Verification items for the finished model (mm, model axes). Face numbers are marked on the shaded views. A direction names the side the tool comes from. Give positions to 0.01 mm unless a question says otherwise; leave off trailing zeros. Write each loop counter-clockwise with the first axis right and the second up, starting at its lowest first coordinate (ties: lowest second). Pieces come first, ordered by that corner, then holes. Notation, with made-up numbers: (79.25, 80.25) -> (117.25, 80.25) arc R14 ccw to (117.25, 104.25) -> close; hole circle Ø10 at (-29.5, 52). An arc over 180 degrees is marked (long way). Answer as CSV lines item,"result". Start each with the question number.
1) Sectioned sample at A-A on y = 0. Give the number of separate pieces and of enclosed holes in the cut face, and give its area (3 significant figures).
2) Gauge pin test, flat ends, axial feed: pin 1 Ø3 at (x, z) = (-98, 45.5) entering from +Y; pin 2 Ø2.5 at (y, z) = (-0.5, 28) entering from +X; pin 3 Ø1.5 at (y, z) = (-4.5, 22.5) entering from +X; pin 4 Ø18.5 at (x, z) = (-110, 33) entering from -Y. Record the tip position at first contact, or that the pin passes through.
3) Sectioned sample at B-B on x = 0. Record the cut outline in (y, z).
4) Mould release check, pull along Z, two halves, no side actions. Record for the marked faces 1 and 2: released by +Z, released by -Z, zero draft, split by the parting line, or undercut.
5) Sectioned sample at D-D on z = 58. Record the cut outline in (x, y), and give its area (3 significant figures).
6) Material ranges on L1, parallel to X at y = 2, z = 34.5; L2, parallel to X at y = -1.5, z = 34.5; L3, parallel to Z at x = -29.5, y = -1.25, recorded low to high.
7) Tool access check on the marked faces 3, 4, 5 and 6. Record the directions out of +Z, -Z, +X, -X, +Y, -Y that give a thin tool (end or side, any length) a straight path to the whole face; none if there is none.
```python
from build123d import *

# Parameters (mm, degrees)
SKETCH1_R           = 6.35
SKETCH1_R_2         = 3.175
BOSS_EXTRUDE1_DEPTH = 62.992
SKETCH3_R           = 3.175
SKETCH6_W           = 22.86
SKETCH6_H           = 1.5875
BOSS_EXTRUDE3_DEPTH = 29.21
SKETCH7_R           = 4.7625
CUT_EXTRUDE1_DEPTH  = 29.21
SKETCH9_R           = 6.35
SKETCH9_R_2         = 3.175
BOSS_EXTRUDE5_DEPTH = 6.35
SKETCH10_R          = 6.35
SKETCH10_R_2        = 5.55625
CUT_EXTRUDE6_DEPTH  = 12.7
SKETCH12_R          = 6.35
SKETCH12_R_2        = 5.55625
CUT_EXTRUDE7_DEPTH  = 12.7
SKETCH13_R          = 5.55625
SKETCH13_R_2        = 3.175
CUT_EXTRUDE8_DEPTH  = 6.35
SKETCH14_R          = 5.55625
SKETCH14_R_2        = 3.175
CUT_EXTRUDE9_DEPTH  = 6.35
SKETCH16_R          = 3.96875
CUT_EXTRUDE11_DEPTH = 142.896915114
SKETCH18_R          = 5.55625
SKETCH18_R_2        = 3.96875
BOSS_EXTRUDE7_DEPTH = 0.508


with BuildPart() as part:
    # Sketch1 → Boss-Extrude1 (new body)
    with BuildSketch(Plane.XY):
        Circle(SKETCH1_R)
        Circle(SKETCH1_R_2, mode=Mode.SUBTRACT)
    extrude(amount=BOSS_EXTRUDE1_DEPTH)

    # Sweep1: sweep along a path in Sketch4
    with BuildLine(Plane(origin=(0, 0, 0), x_dir=(1, 0, 0), z_dir=(0, 1, 0))) as sweep1_path:
        Line((-3.81, -15.663931971), (-107.95, -15.663931971))
        ThreePointArc((-107.95, -15.663931971), (-123.665226198, -31.37915817), (-107.95, -47.094384368))
        Line((-107.95, -47.094384368), (-3.81, -47.094384368))
    # Sketch3 → Sweep1 (sweep)
    with BuildSketch(Plane.ZY.offset(3.81)):
        with Locations((47.244, 0)):
            Circle(SKETCH3_R)
    sweep(path=sweep1_path.line)

    # Sketch6 → Boss-Extrude3 (add)
    with BuildSketch(Plane.XY.offset(15.24)):
        with Locations((-105.071320577, -0.79375)):
            Rectangle(SKETCH6_W, SKETCH6_H)
        with Locations((-105.071320577, 0.79375)):
            Rectangle(SKETCH6_W, SKETCH6_H)
    extrude(amount=BOSS_EXTRUDE3_DEPTH)

    # Sketch7 → Cut-Extrude1 (cut)
    with BuildSketch(Plane(origin=(0, 1.5875, 0), x_dir=(1, 0, 0), z_dir=(0, 1, 0))):
        with Locations(Location((-105.071320577, -31.341130791, 0), (0, 0, 180))):
            Circle(SKETCH7_R)
    extrude(amount=-CUT_EXTRUDE1_DEPTH, mode=Mode.SUBTRACT)

    # Sketch9 → Boss-Extrude5 (add)
    with BuildSketch(Plane(origin=(0, 0, 0), x_dir=(-1, 0, 0), z_dir=(0, 0, -1))):
        Circle(SKETCH9_R)
        Circle(SKETCH9_R_2, mode=Mode.SUBTRACT)
    boss_extrude5 = extrude(amount=BOSS_EXTRUDE5_DEPTH)

    # Mirror1: Boss-Extrude5 across plane
    add(boss_extrude5.mirror(Plane.XY.offset(31.496)))

    # Sketch10 → Cut-Extrude6 (cut)
    with BuildSketch(Plane.XY.offset(69.342)):
        with Locations(Location((0, 0, 0), (0, 0, 180))):
            Circle(SKETCH10_R)
        with Locations(Location((0, 0, 0), (0, 0, 180))):
            Circle(SKETCH10_R_2, mode=Mode.SUBTRACT)
    extrude(amount=-CUT_EXTRUDE6_DEPTH, mode=Mode.SUBTRACT)

    # Sketch12 → Cut-Extrude7 (cut)
    with BuildSketch(Plane(origin=(0, 0, -6.35), x_dir=(-1, 0, 0), z_dir=(0, 0, -1))):
        Circle(SKETCH12_R)
        Circle(SKETCH12_R_2, mode=Mode.SUBTRACT)
    extrude(amount=-CUT_EXTRUDE7_DEPTH, mode=Mode.SUBTRACT)

    # Sketch13 → Cut-Extrude8 (cut)
    with BuildSketch(Plane.XY.offset(69.342)):
        with Locations(Location((0, 0, 0), (0, 0, 180))):
            Circle(SKETCH13_R)
        Circle(SKETCH13_R_2, mode=Mode.SUBTRACT)
    extrude(amount=-CUT_EXTRUDE8_DEPTH, mode=Mode.SUBTRACT)

    # Sketch14 → Cut-Extrude9 (cut)
    with BuildSketch(Plane(origin=(0, 0, -6.35), x_dir=(-1, 0, 0), z_dir=(0, 0, -1))):
        Circle(SKETCH14_R)
        Circle(SKETCH14_R_2, mode=Mode.SUBTRACT)
    extrude(amount=-CUT_EXTRUDE9_DEPTH, mode=Mode.SUBTRACT)

    # Sketch16 → Cut-Extrude11 (cut, through all)
    with BuildSketch(Plane(origin=(0, 0, 0), x_dir=(-1, 0, 0), z_dir=(0, 0, -1))):
        Circle(SKETCH16_R)
    extrude(amount=-CUT_EXTRUDE11_DEPTH, mode=Mode.SUBTRACT)

    # Sketch18 → Boss-Extrude7 (add)
    with BuildSketch(Plane(origin=(0, 0, 0), x_dir=(-1, 0, 0), z_dir=(0, 0, -1))):
        Circle(SKETCH18_R)
        Circle(SKETCH18_R_2, mode=Mode.SUBTRACT)
    extrude(amount=BOSS_EXTRUDE7_DEPTH)


solid = part.part
```
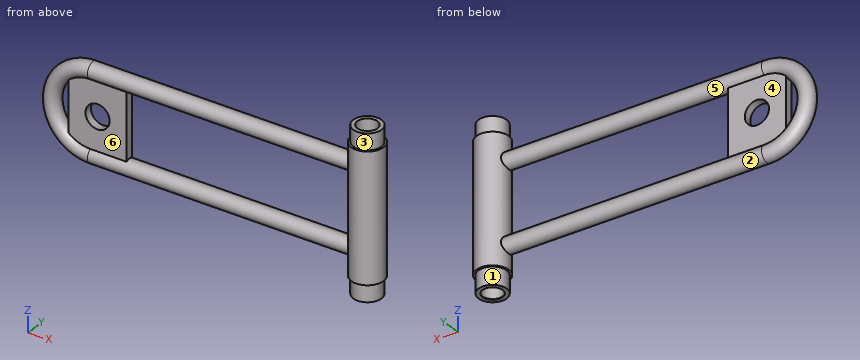
Ans:
1,separate pieces,"2"
1,enclosed holes,"3"
1,area,"2,380 mm²"
2,pin 1,"stops at y = 3.17"
2,pin 2,"stops at x = 6.35"
2,pin 3,"stops at x = 5.12"
2,pin 4,"stops at y = -1.59"
3,outline,"(-6.35, 6.35) -> (-5.56, 6.35) -> (-5.56, -0.51) -> (-3.97, -0.51) -> (-3.97, 62.99) -> (-5.56, 62.99) -> (-5.56, 56.64) -> (-6.35, 56.64) -> close; (3.97, -0.51) -> (5.56, -0.51) -> (5.56, 6.35) -> (6.35, 6.35) -> (6.35, 56.64) -> (5.56, 56.64) -> (5.56, 62.99) -> (3.97, 62.99) -> close"
4,face 1,"zero draft"
4,face 2,"undercut"
5,outline,"circle Ø11.11 at (0, 0); hole circle Ø7.94 at (0, 0)"
5,area,"47.5 mm²"
6,L1,"x = -126.01 to -120.98, -6.03 to -3.43, 3.43 to 6.03"
6,L2,"x = -126.35 to -120.64, -116.5 to -108.64, -101.51 to -93.64, -6.17 to -3.67, 3.67 to 6.17"
6,L3,"z = 12.6 to 18.43, 44.33 to 50.16"
7,face 3,"+Z"
7,face 4,"+Y"
7,face 5,"none"
7,face 6,"-Y"
